The listing builds one solid part. Answer for the finished solid, in the listing's coordinates (mm). Coordinates: 2 decimals unless noted, no trailing zeros. Order: outer loops, then holes, each group sorted by start corner. A loop starts at its lowest first (then second) coordinate and runs counter-clockwise, first axis right, second up.
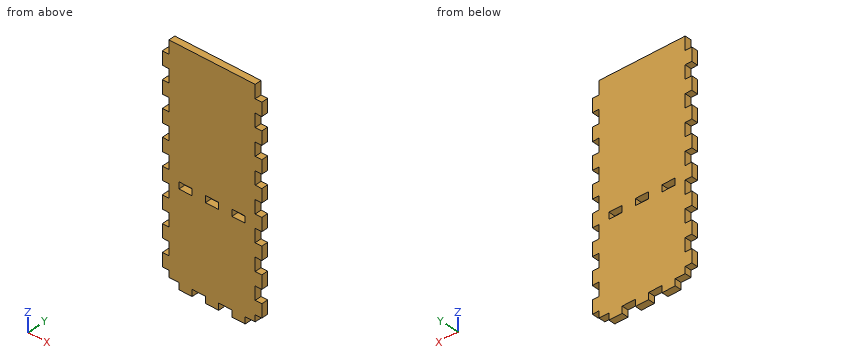
```python
from build123d import *

# Parameters (mm, degrees)
SKETCH1_W           = 95.25
SKETCH1_H           = 215.9
BOSS_EXTRUDE1_DEPTH = 6.35
SKETCH2_W           = 6.35
SKETCH2_H           = 12.7
CUT_EXTRUDE1_DEPTH  = 7.35
LPATTERN1_COUNT     = 10
LPATTERN1_PITCH     = 25.4
SKETCH3_W           = 12.7
SKETCH3_H           = 6.35
CUT_EXTRUDE2_DEPTH  = 7.35
LPATTERN2_COUNT     = 2
LPATTERN2_PITCH     = 25.4
LPATTERN2_COL_COUNT = 3
LPATTERN2_COL_PITCH = 25.4
SKETCH4_W           = 12.7
SKETCH4_H           = 6.35
CUT_EXTRUDE3_DEPTH  = 7.35


with BuildPart() as part:
    # Sketch1 → Boss-Extrude1 (new body)
    with BuildSketch(Plane(origin=(0, 0, 0), x_dir=(1, 0, 0), z_dir=(0, 1, 0))):
        with Locations((47.625, 107.95)):
            Rectangle(SKETCH1_W, SKETCH1_H)
    extrude(amount=BOSS_EXTRUDE1_DEPTH)

    # Sketch2 → Cut-Extrude1 (cut, through all)
    with BuildSketch(Plane(origin=(0, 6.35, 0), x_dir=(1, 0, 0), z_dir=(0, 1, 0))):
        with Locations((3.175, 209.55)):
            Rectangle(SKETCH2_W, SKETCH2_H)
        with Locations((92.075, 209.55)):
            Rectangle(SKETCH2_W, SKETCH2_H)
    cut_extrude1 = extrude(amount=-CUT_EXTRUDE1_DEPTH, mode=Mode.SUBTRACT)

    # LPattern1: Cut-Extrude1 ×10
    with Locations(*[(0, 0, i * LPATTERN1_PITCH) for i in range(1, LPATTERN1_COUNT)]):
        add(cut_extrude1, mode=Mode.SUBTRACT)

    # Sketch3 → Cut-Extrude2 (cut, through all)
    with BuildSketch(Plane(origin=(0, 6.35, 0), x_dir=(1, 0, 0), z_dir=(0, 1, 0))):
        with Locations((34.925, 212.725)):
            Rectangle(SKETCH3_W, SKETCH3_H)
    cut_extrude2 = extrude(amount=-CUT_EXTRUDE2_DEPTH, mode=Mode.SUBTRACT)

    # LPattern2: Cut-Extrude2 ×2
    with Locations(*[(-i * LPATTERN2_PITCH, 0, 0) for i in range(1, LPATTERN2_COUNT)]):
        add(cut_extrude2, mode=Mode.SUBTRACT)

    # LPattern2 col: Cut-Extrude2 ×3
    with Locations(*[(i * LPATTERN2_COL_PITCH, 0, 0) for i in range(1, LPATTERN2_COL_COUNT)]):
        add(cut_extrude2, mode=Mode.SUBTRACT)

    # Sketch4 → Cut-Extrude3 (cut, through all)
    with BuildSketch(Plane(origin=(0, 6.35, 0), x_dir=(1, 0, 0), z_dir=(0, 1, 0))):
        with Locations((22.225, 123.825)):
            Rectangle(SKETCH4_W, SKETCH4_H)
        with Locations((47.625, 123.825)):
            Rectangle(SKETCH4_W, SKETCH4_H)
        with Locations((73.025, 123.825)):
            Rectangle(SKETCH4_W, SKETCH4_H)
    extrude(amount=-CUT_EXTRUDE3_DEPTH, mode=Mode.SUBTRACT)


solid = part.part
```
(1) Find section C-C (x = 38). Write down the section's boundary in (y, z).
(2) Consider line 1 (Z direction, x = 19.5, y = 5.75); line 2 (Z direction, x = 65, y = 4); line 3 (X direction, y = 2, z = -29). Determine where each line is inside the solid, lowest interval first.
(3) Each of these flat-tipped pins is pushed along its axis until it touches: pin 1 Ø1.9 at (x, y) = (92, 2.5) entering from +Z; pin 2 Ø3 at (y, z) = (4, -83.5) entering from -X; pin 3 Ø2 at (x, z) = (23.5, -56) entering from -Y; pin 4 Ø1.9 at (x, y) = (4.5, 3) entering from -Z. Where does it stop, or does it pass through?
(4) Find section A-A (x = 74). Write down the section's boundary in (y, z), and give its area (3 significant figures).
(5) Find section B-B (y = 4.5). Give the number of separate pieces and of enclosed holes in the cut face, and give its area (3 significant figures).
Findings below:
1. outline: (0, -209.55) - (6.35, -209.55) - (6.35, 0) - (0, 0) - close
2. line 1: z = -215.9 to -127, -120.65 to 0
2. line 2: z = -209.55 to 0
2. line 3: x = 6.35 to 88.9
3. pin 1: stops at z = -12.7
3. pin 2: stops at x = 6.35
3. pin 3: stops at y = 0
3. pin 4: stops at z = -203.2
4. outline: (0, -215.9) - (6.35, -215.9) - (6.35, -127) - (0, -127) - close; (0, -120.65) - (6.35, -120.65) - (6.35, 0) - (0, 0) - close
4. area: 1,330 mm2
5. separate pieces: 1
5. enclosed holes: 3
5. area: 18,600 mm2
